```python
from build123d import *

# Parameters (mm, degrees)
BOSS_EXTRUDE1_DEPTH = 10
SKETCH2_W           = 5.8
SKETCH2_H           = 3.8
BOSS_EXTRUDE2_DEPTH = 2
SKETCH3_R           = 2.15
CUT_EXTRUDE1_DEPTH  = 12
CUT_EXTRUDE5_START  = -10
SKETCH4_W           = 7.6
SKETCH4_H           = 3.5
CUT_EXTRUDE5_DEPTH  = 8.75
SKETCH7_W           = 7.6
SKETCH7_H           = 3.5
CUT_EXTRUDE6_DEPTH  = 8.75
CUT_EXTRUDE7_DEPTH  = 8.75
SKETCH12_R          = 2.5
CUT_EXTRUDE8_DEPTH  = 10


with BuildPart() as part:
    # Sketch1 → Boss-Extrude1 (new body)
    with BuildSketch(Plane.XY):
        Polygon((0, 70.768728377), (0, 0), (33, 0), align=None)
    extrude(amount=BOSS_EXTRUDE1_DEPTH)

    # Sketch2 → Boss-Extrude2 (add)
    with BuildSketch(Plane(origin=(0, 0, 0), x_dir=(-1, 0, 0), z_dir=(0, -1, 0))):
        with Locations((-16.5, -5)):
            Rectangle(SKETCH2_W, SKETCH2_H)
    extrude(amount=BOSS_EXTRUDE2_DEPTH)

    # Sketch3 → Cut-Extrude1 (cut)
    with BuildSketch(Plane(origin=(0, 0, 0), x_dir=(-1, 0, 0), z_dir=(0, -1, 0))):
        with Locations(Location((-23.33, -6, 0), (0, 0, 180))):
            Circle(SKETCH3_R)
        with Locations(Location((-8.55, -6, 0), (0, 0, 180))):
            Circle(SKETCH3_R)
    extrude(amount=-CUT_EXTRUDE1_DEPTH, mode=Mode.SUBTRACT)

    # Sketch4 → Cut-Extrude5 (cut)
    with BuildSketch(Plane(origin=(0, 0, 0), x_dir=(-1, 0, 0), z_dir=(0, 0, -1)).offset(CUT_EXTRUDE5_START)):
        with Locations((-23.33, 5.001728642)):
            Rectangle(SKETCH4_W, SKETCH4_H)
    extrude(amount=CUT_EXTRUDE5_DEPTH, mode=Mode.SUBTRACT)

    # Sketch7 → Cut-Extrude6 (cut)
    with BuildSketch(Plane.XY.offset(10)):
        with Locations((8.567911565, 5.001728642)):
            Rectangle(SKETCH7_W, SKETCH7_H)
    extrude(amount=-CUT_EXTRUDE6_DEPTH, mode=Mode.SUBTRACT)

    # Sketch10 → Cut-Extrude7 (cut)
    with BuildSketch(Plane.XY.offset(10)):
        Polygon((6.237191143, 40.829617725), (9.862422291, 42.520090772), (8.256472896, 45.964060362), (4.631241748, 44.273587315), align=None)
        Polygon((11.468371686, 39.076121181), (9.862422291, 42.520090772), (6.237191143, 40.829617725), (7.843140537, 37.385648134), align=None)
        Polygon((17.386162964, 12.927131096), (21.011394112, 14.617604143), (19.405444717, 18.061573734), (15.780213569, 16.371100687), align=None)
        Polygon((22.617343506, 11.173634553), (21.011394112, 14.617604143), (17.386162964, 12.927131096), (18.992112358, 9.483161506), align=None)
    extrude(amount=-CUT_EXTRUDE7_DEPTH, mode=Mode.SUBTRACT)

    # Sketch12 → Cut-Extrude8 (cut)
    with BuildSketch(Plane(origin=(27.10599556, 12.639733311, 0), x_dir=(0, 0, -1), z_dir=(0.9063077870366479, 0.422618261740704, 0))):
        with Locations(Location((-5, 34.368249607, 0), (0, 0, 90))):
            Circle(SKETCH12_R)
        with Locations(Location((-5, 4.368249607, 0), (0, 0, 90))):
            Circle(SKETCH12_R)
    extrude(amount=-CUT_EXTRUDE8_DEPTH, mode=Mode.SUBTRACT)


solid = part.part
```
Design review of the part built by this model. Coordinates are the model's own, in mm. A direction names the side the tool comes from. Coordinates: 2 decimals unless noted, no trailing zeros. Order: outer loops, then holes, each group sorted by start corner. A loop starts at its lowest first (then second) coordinate and runs counter-clockwise, first axis right, second up. Notation, with made-up numbers: (2.5, 2) - (40.5, 2) arc R23 cw to (40.5, 27) - close; hole circle Ø11 at (76.5, 24). An arc over 180 degrees is marked (long way). Answer in a Markdown table with one row per item.
(1) Wall thickness on line 1 along Z through (x, y) = (23.33, 10.55); line 2 along Y through (x, z) = (21, 5); line 3 along Y through (x, z) = (5, 7.75): over which ranges is each line inside the solid? List them lowest first. Write a range as from..to.
Checked values:
| item | result |
|---|---|
| line 1 | 0..3.85, 8.15..10 |
| line 2 | 0..3.25, 6.75..10.42, 17.37..25.73 |
| line 3 | 0..3.25, 6.75..43.48, 44.45..60.05 |
(2) Consider section C-C on y = 64. State the section outline as (x, z) points, plus the area to 3 significant figures.
Checked values:
| item | result |
|---|---|
| outline | (0, 0) - (3.16, 0) - (3.16, 10) - (0, 10) - close |
| area | 31.6 mm^2 |
(3) The part is to be moulded in two halves that separate along Y. For faces 1 (the cylindrical face through (6.4, 1.6, 6.09)), 2 (the flat face through (16.73, 34.89, 4.93)), 3 (the flat face through (9.63, 38.22, 5.69)), say which applies: released by +Y, released by -Y, zero draft, split by the parting line, or undercut.
Checked values:
| item | result |
|---|---|
| face 1 | zero draft |
| face 2 | released by +Y |
| face 3 | undercut |
(4) Clearance check with flat-ended pins moving along their axes: pin 1 (1.5 mm diameter, centred on x = 13, z = 7, fed in from -Y); pin 2 (1 mm diameter, centred on x = 16, y = -1, fed in from -Z); pin 3 (2 mm diameter, centred on x = 8, z = 6.5, fed in from -Y); pin 4 (6 mm diameter, centred on x = 21.5, z = 7, fed in from +Y). State where each tip first meets the part, or that it passes through.
Checked values:
| item | result |
|---|---|
| pin 1 | y = -2 |
| pin 2 | z = 3.1 |
| pin 3 | y = 12 |
| pin 4 | y = 31.1 |
(5) For faces 4 (the flat face through (3.533, 39.53, 5.035)), 5 (the flat face through (17.62, 17.23, 5.69)), 6 (the cylindrical face through (25.38, 9.34, 6.65)), 7 (the flat face through (17, -1, 3.1)), 8 (the flat face through (13.6, -1, 5)), list the 3-axis set-ups (+Z, -Z, +X, -X, +Y, -Y) from which the entire face can be reached by the end or side of a thin tool; tool diameter is ignored.
Checked values:
| item | result |
|---|---|
| face 4 | none |
| face 5 | +Z |
| face 6 | -Y |
| face 7 | -Z, +X, -X, -Y |
| face 8 | +Z, -Z, -X, -Y |
(6) Consider section A-A on x = 23.33. Give the number of separate pieces and of enclosed holes in the cut face, plus the area to 3 significant figures.
Checked values:
| item | result |
|---|---|
| separate pieces | 2 |
| enclosed holes | 1 |
| area | 119 mm^2 |
(7) Consider section B-B on y = 50.5. State the section outline as (x, z) points.
Checked values:
| item | result |
|---|---|
| outline | (0, 0) - (9.45, 0) - (9.45, 10) - (0, 10) - close |
